Input: part model. Units: mm. Frame: model coordinates. Face numbers are marked on the shaded views. A direction names the side the tool comes from. Give positions to 0.01 mm unless a question says otherwise; leave off trailing zeros. Order: outer loops, then holes, each group sorted by start corner. A loop starts at its lowest first (then second) coordinate and runs counter-clockwise, first axis right, second up. Notation, with made-up numbers: (-6, 71.5) - (28, 71.5) arc R29 cw to (28, 97.5) - close; hole circle Ø10 at (74.25, -17.5). An arc over 180 degrees is marked (long way). Use a Markdown table: item, result.
from build123d import *

# Parameters (mm, degrees)
PAD_DEPTH    = 42
POCKET_DEPTH = 40
PAD001_DEPTH = 6
PAD002_DEPTH = 5


with BuildPart() as part:
    # Sketch → Pad (new body)
    with BuildSketch(Plane.XY):
        with BuildLine():
            Line((-91.5, 36.5), (-91.5, -36.5))
            ThreePointArc((-91.5, -36.5), (-88.571068, -43.571068), (-81.5, -46.5))
            Line((-81.5, -46.5), (81.5, -46.5))
            ThreePointArc((81.5, -46.5), (88.571068, -43.571068), (91.5, -36.5))
            Line((91.5, -36.5), (91.5, 36.5))
            ThreePointArc((91.5, 36.5), (88.571068, 43.571068), (81.5, 46.5))
            Line((81.5, 46.5), (-81.5, 46.5))
            ThreePointArc((-81.5, 46.5), (-88.571068, 43.571068), (-91.5, 36.5))
        make_face()
    extrude(amount=PAD_DEPTH)

    # Sketch001 (on Face10 of Pad) → Pocket (cut)
    with BuildSketch(Plane.XY.offset(42)):
        with BuildLine():
            Line((-90, 35), (-90, -35))
            ThreePointArc((-90, -35), (-87.071068, -42.071068), (-80, -45))
            Line((-80, -45), (80, -45))
            ThreePointArc((80, -45), (87.071068, -42.071068), (90, -35))
            Line((90, -35), (90, 35))
            ThreePointArc((90, 35), (87.071068, 42.071068), (80, 45))
            Line((80, 45), (-80, 45))
            ThreePointArc((-80, 45), (-87.071068, 42.071068), (-90, 35))
        make_face()
    extrude(amount=-POCKET_DEPTH, mode=Mode.SUBTRACT)

    # Sketch002 (on Face6 of Pocket) → Pad001 (join)
    with BuildSketch(Plane(origin=(0, 46.5, 0), x_dir=(-1, 0, 0), z_dir=(0, 1, 0))):
        with BuildLine():
            ThreePointArc((-17.8, 30.8), (-20, 33), (-22.2, 30.8))
            Line((-22.2, 30.8), (-22.2, 28.7))
            ThreePointArc((-22.2, 28.7), (-20, 26.5), (-17.8, 28.7))
            Line((-17.8, 30.8), (-17.8, 28.7))
        make_face()
        with BuildLine():
            ThreePointArc((22.2, 30.8), (20, 33), (17.8, 30.8))
            Line((17.8, 30.8), (17.8, 28.7))
            ThreePointArc((17.8, 28.7), (20, 26.5), (22.2, 28.7))
            Line((22.2, 30.8), (22.2, 28.7))
        make_face()
        with BuildLine():
            ThreePointArc((62.2, 30.8), (60, 33), (57.8, 30.8))
            Line((57.8, 30.8), (57.8, 28.7))
            ThreePointArc((57.8, 28.7), (60, 26.5), (62.2, 28.7))
            Line((62.2, 30.8), (62.2, 28.7))
        make_face()
        with BuildLine():
            ThreePointArc((-37.8, 10.8), (-40, 13), (-42.2, 10.8))
            Line((-42.2, 10.8), (-42.2, 8.7))
            ThreePointArc((-42.2, 8.7), (-40, 6.5), (-37.8, 8.7))
            Line((-37.8, 10.8), (-37.8, 8.7))
        make_face()
        with BuildLine():
            ThreePointArc((2.2, 10.8), (0, 13), (-2.2, 10.8))
            Line((-2.2, 10.8), (-2.2, 8.7))
            ThreePointArc((-2.2, 8.7), (0, 6.5), (2.2, 8.7))
            Line((2.2, 10.8), (2.2, 8.7))
        make_face()
        with BuildLine():
            ThreePointArc((42.2, 10.8), (40, 13), (37.8, 10.8))
            Line((37.8, 10.8), (37.8, 8.7))
            ThreePointArc((37.8, 8.7), (40, 6.5), (42.2, 8.7))
            Line((42.2, 10.8), (42.2, 8.7))
        make_face()
        with BuildLine():
            ThreePointArc((-57.8, 30.8), (-60, 33), (-62.2, 30.8))
            Line((-62.2, 30.8), (-62.2, 28.7))
            ThreePointArc((-62.2, 28.7), (-60, 26.5), (-57.8, 28.7))
            Line((-57.8, 30.8), (-57.8, 28.7))
        make_face()
    extrude(amount=PAD001_DEPTH)

    # Sketch003 (on Face49 of Pad001) → Pad002 (join)
    with BuildSketch(Plane(origin=(0, 52.5, 0), x_dir=(-1, 0, 0), z_dir=(0, 1, 0))):
        with BuildLine():
            ThreePointArc((62.2, 30.8), (60, 33), (57.8, 30.8))
            Line((57.8, 30.8), (57.8, 22.2))
            ThreePointArc((57.8, 22.2), (60, 20), (62.2, 22.2))
            Line((62.2, 30.8), (62.2, 22.2))
        make_face()
        with BuildLine():
            ThreePointArc((22.2, 30.8), (20, 33), (17.8, 30.8))
            Line((17.8, 30.8), (17.8, 22.2))
            ThreePointArc((17.8, 22.2), (20, 20), (22.2, 22.2))
            Line((22.2, 30.8), (22.2, 22.2))
        make_face()
        with BuildLine():
            ThreePointArc((42.2, 10.8), (40, 13), (37.8, 10.8))
            Line((37.8, 10.8), (37.8, 2.2))
            ThreePointArc((37.8, 2.2), (40, 0), (42.2, 2.2))
            Line((42.2, 10.8), (42.2, 2.2))
        make_face()
        with BuildLine():
            ThreePointArc((-17.8, 30.8), (-20, 33), (-22.2, 30.8))
            Line((-22.2, 30.8), (-22.2, 22.2))
            ThreePointArc((-22.2, 22.2), (-20, 20), (-17.8, 22.2))
            Line((-17.8, 30.8), (-17.8, 22.2))
        make_face()
        with BuildLine():
            ThreePointArc((2.2, 10.8), (0, 13), (-2.2, 10.8))
            Line((-2.2, 10.8), (-2.2, 2.2))
            ThreePointArc((-2.2, 2.2), (0, 0), (2.2, 2.2))
            Line((2.2, 10.8), (2.2, 2.2))
        make_face()
        with BuildLine():
            ThreePointArc((-37.8, 10.8), (-40, 13), (-42.2, 10.8))
            Line((-42.2, 10.8), (-42.2, 2.2))
            ThreePointArc((-42.2, 2.2), (-40, 0), (-37.8, 2.2))
            Line((-37.8, 10.8), (-37.8, 2.2))
        make_face()
        with BuildLine():
            ThreePointArc((-57.8, 30.8), (-60, 33), (-62.2, 30.8))
            Line((-62.2, 30.8), (-62.2, 22.2))
            ThreePointArc((-62.2, 22.2), (-60, 20), (-57.8, 22.2))
            Line((-57.8, 30.8), (-57.8, 22.2))
        make_face()
    extrude(amount=PAD002_DEPTH)


solid = part.part
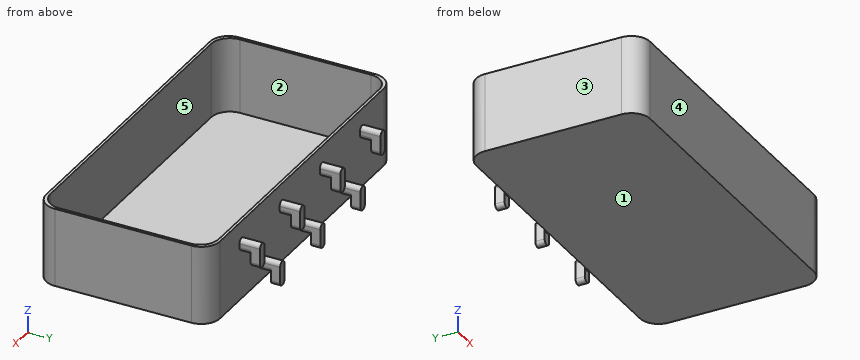
1. Section query B-B (y = -6.5). Return loops of the section in (x, z), then the cut area to 3 significant figures.
Response:
| item | result |
|---|---|
| outline | (-91.5, 0) - (91.5, 0) - (91.5, 42) - (90, 42) - (90, 2) - (-90, 2) - (-90, 42) - (-91.5, 42) - close |
| area | 486 mm^2 |
2. Section query A-A (x = -40). Return loops of the section in (y, z), then the cut area to 3 significant figures.
Response:
| item | result |
|---|---|
| outline | (-46.5, 0) - (46.5, 0) - (46.5, 6.5) - (52.5, 6.5) - (52.5, 0) - (57.5, 0) - (57.5, 13) - (46.5, 13) - (46.5, 42) - (45, 42) - (45, 2) - (-45, 2) - (-45, 42) - (-46.5, 42) - close |
| area | 410 mm^2 |
3. Material intervals for line 1 along X through (y, z) = (-3, 31.5); line 2 along Y through (x, z) = (56, 34.5); line 3 along Z through (x, y) = (-48, 13.5), sorted ascending.
Response:
| item | result |
|---|---|
| line 1 | x = -91.5 to -90, 90 to 91.5 |
| line 2 | y = -46.5 to -45, 45 to 46.5 |
| line 3 | z = 0 to 2 |
4. Mould query, pull axis Y, two halves, no side actions, for the marked faces 3, 4 and 5. Classes: pulls with the +Y half, pulls with the -Y half, needs draft (parallel to the pull), parting line crosses it, or undercut.
Response:
| item | result |
|---|---|
| face 3 | needs draft |
| face 4 | pulls with the -Y half |
| face 5 | undercut |
5. Set-up query: the marked faces 1 and 2. Return all of +Z, -Z, +X, -X, +Y, -Y with unobstructed straight access to the full face (end or side cutting, diameter ignored); none if empty.
Response:
| item | result |
|---|---|
| face 1 | -Z, +X, -X, +Y, -Y |
| face 2 | +Z |
6. Pin query (flat end, axial travel): pin 1 (2.5 mm diameter, centred on y = 49.5, z = 8.5, fed in from -X); pin 2 (4 mm diameter, centred on x = -2.5, z = 18.5, fed in from +Y); pin 3 (9.5 mm diameter, centred on y = 50, z = 25.5, fed in from +X). Return the tip coordinate at first contact, or that it passes through.
Response:
| item | result |
|---|---|
| pin 1 | stops at x = -42.2 |
| pin 2 | stops at y = 46.5 |
| pin 3 | stops at x = 86.34 |
